Work out the finished part from the listing and answer in its coordinate system (mm). A direction names the side the tool comes from. Coordinates: 2 decimals unless noted, no trailing zeros. Order: outer loops, then holes, each group sorted by start corner. A loop starts at its lowest first (then second) coordinate and runs counter-clockwise, first axis right, second up. Notation, with made-up numbers: M 20.5,78.25 L 40.5,78.25 A23 cw 40.5,96.25 Z; hole C 83,67.5 d2. An arc over 180 degrees is marked long. Use a Markdown table: item, result.
from build123d import *

# Parameters (mm, degrees)
SALIENTE_EXTRUIR2_DEPTH = 50
CROQUIS3_R              = 5
CORTAR_EXTRUIR3_DEPTH   = 10
CROQUIS5_W              = 26
CROQUIS5_H              = 20
CORTAR_EXTRUIR4_DEPTH   = 100


with BuildPart() as part:
    # Croquis1 → Saliente-Extruir2 (new body)
    with BuildSketch(Plane.XY):
        with BuildLine():
            Line((-68.920564692, -21.589574482), (-23.920564692, -21.589574482))
            ThreePointArc((-23.920564692, -21.589574482), (-3.920564692, -1.589574482), (16.079435308, -21.589574482))
            Line((16.079435308, -21.589574482), (21.079435308, -21.589574482))
            Line((21.079435308, -21.589574482), (21.079435308, 28.410425518))
            Line((21.079435308, 28.410425518), (-3.920564692, 28.410425518))
            Line((-3.920564692, 28.410425518), (-38.920564692, -1.589574482))
            Line((-38.920564692, -1.589574482), (-38.920564692, -11.589574482))
            Line((-38.920564692, -11.589574482), (-68.920564692, -11.589574482))
            Line((-68.920564692, -11.589574482), (-68.920564692, -21.589574482))
        make_face()
    extrude(amount=-SALIENTE_EXTRUIR2_DEPTH)

    # Croquis3 → Cortar-Extruir3 (cut)
    with BuildSketch(Plane(origin=(0, -11.589574482, 0), x_dir=(1, 0, 0), z_dir=(0, 1, 0))):
        with Locations((-54.712100966, 38)):
            Circle(CROQUIS3_R)
        with Locations((-54.712100966, 12)):
            Circle(CROQUIS3_R)
    extrude(amount=-CORTAR_EXTRUIR3_DEPTH, mode=Mode.SUBTRACT)

    # Croquis5 → Cortar-Extruir4 (cut)
    with BuildSketch(Plane(origin=(21.079435308, 0, 0), x_dir=(0, 0, -1), z_dir=(1, 0, 0))):
        with Locations((25, 18.410425518)):
            Rectangle(CROQUIS5_W, CROQUIS5_H)
    extrude(amount=-CORTAR_EXTRUIR4_DEPTH, mode=Mode.SUBTRACT)


solid = part.part
1. Flat-ended cylindrical pins translate along their axes: P1, Ø4, axis at x = 2.5, z = -14.5, coming from the -Y side; P2, Ø2, axis at y = 21.5, z = -44.5, coming from the -X side; P3, Ø13, axis at x = -54.71, z = -12, coming from the +Y side; P4, Ø6, axis at x = -9.5, y = 15, coming from the +Z side. Find the tip coordinate at first contact, or state that the pin passes through.
Answers below:
| item | result |
|---|---|
| P1 | y = -3.45 |
| P2 | x = -13.15 |
| P3 | y = -11.59 |
| P4 | z = 0 |
2. For faces 5 (the face through (-3, 8.41, -25)), 6 (the face through (-47, -21.59, -25)), 7 (the face through (-38.921, -7, -25)), determine the directions among +Z, -Z, +X, -X, +Y, -Y from which every point of the face is accessible in a straight line to the end or side of a thin tool.
Answers below:
| item | result |
|---|---|
| face 5 | +X, -X, +Y |
| face 6 | +Z, -Z, +X, -X, -Y |
| face 7 | +Z, -Z, -X, +Y |
3. Section B-B on y = -15.5 is taken. Determine the outline of the cut face in (x, z).
Answers below:
| item | result |
|---|---|
| outline | M -68.92,-50 L -22.97,-50 L -22.97,0 L -68.92,0 Z; M 15.13,-50 L 21.08,-50 L 21.08,0 L 15.13,0 Z; hole C -54.71,-38 d10; hole C -54.71,-12 d10 |
4. Section A-A on z = -40 is taken. Determine the outline of the cut face in (x, y), then the cut area to 3 significant figures.
Answers below:
| item | result |
|---|---|
| outline | M -68.92,-21.59 L -59.29,-21.59 L -59.29,-11.59 L -68.92,-11.59 Z; M -50.13,-21.59 L -23.92,-21.59 A20 cw 16.08,-21.59 L 21.08,-21.59 L 21.08,28.41 L -3.92,28.41 L -38.92,-1.59 L -38.92,-11.59 L -50.13,-11.59 Z |
| area | 2,060 mm² |
5. Find the intervals of material crossed by probe 1 along Z at (x, y) = (6.5, 11.5); probe 2 along X at (y, z) = (-19, -12); probe 3 along X at (y, z) = (-16, -38), in increasing order.
Answers below:
| item | result |
|---|---|
| probe 1 | -50 to -38, -12 to 0 |
| probe 2 | -68.92 to -59.71, -49.71 to -23.75, 15.91 to 21.08 |
| probe 3 | -68.92 to -59.71, -49.71 to -23.12, 15.28 to 21.08 |
6. For a pull along X with two mould halves and no side action, classify faces 1 (the face through (-4.36, -1.594, -24.65)), 2 (the face through (21.079, -2, -25)), 3 (the face through (9, 28.41, -6)), 4 (the face through (-28.953, 6.954, -24.65)) as +X half, -X half, draft (parallel to the pull), parting line (faces both ways), or undercut.
Answers below:
| item | result |
|---|---|
| face 1 | undercut |
| face 2 | +X half |
| face 3 | draft |
| face 4 | -X half |
7. Section D-D on z = -26.5 is taken. Determine the outline of the cut face in (x, y).
Answers below:
| item | result |
|---|---|
| outline | M -68.92,-21.59 L -23.92,-21.59 A20 cw 16.08,-21.59 L 21.08,-21.59 L 21.08,8.41 L -27.25,8.41 L -38.92,-1.59 L -38.92,-11.59 L -68.92,-11.59 Z |
8. Section C-C on y = -10 is taken. Determine the outline of the cut face in (x, z).
Answers below:
| item | result |
|---|---|
| outline | M -38.92,-50 L -20.22,-50 L -20.22,0 L -38.92,0 Z; M 12.38,-50 L 21.08,-50 L 21.08,0 L 12.38,0 Z |
